Answer from the drawing. Dimensions are ordinates in mm from the lowest x, y and z of the part. Give positions to 0.01 mm unless a question says otherwise; leave off trailing zeros. Write each loop counter-clockwise with the first axis right and the second up, starting at its lowest first coordinate (ties: lowest second). Pieces come first, ordered by that corner, then holes.
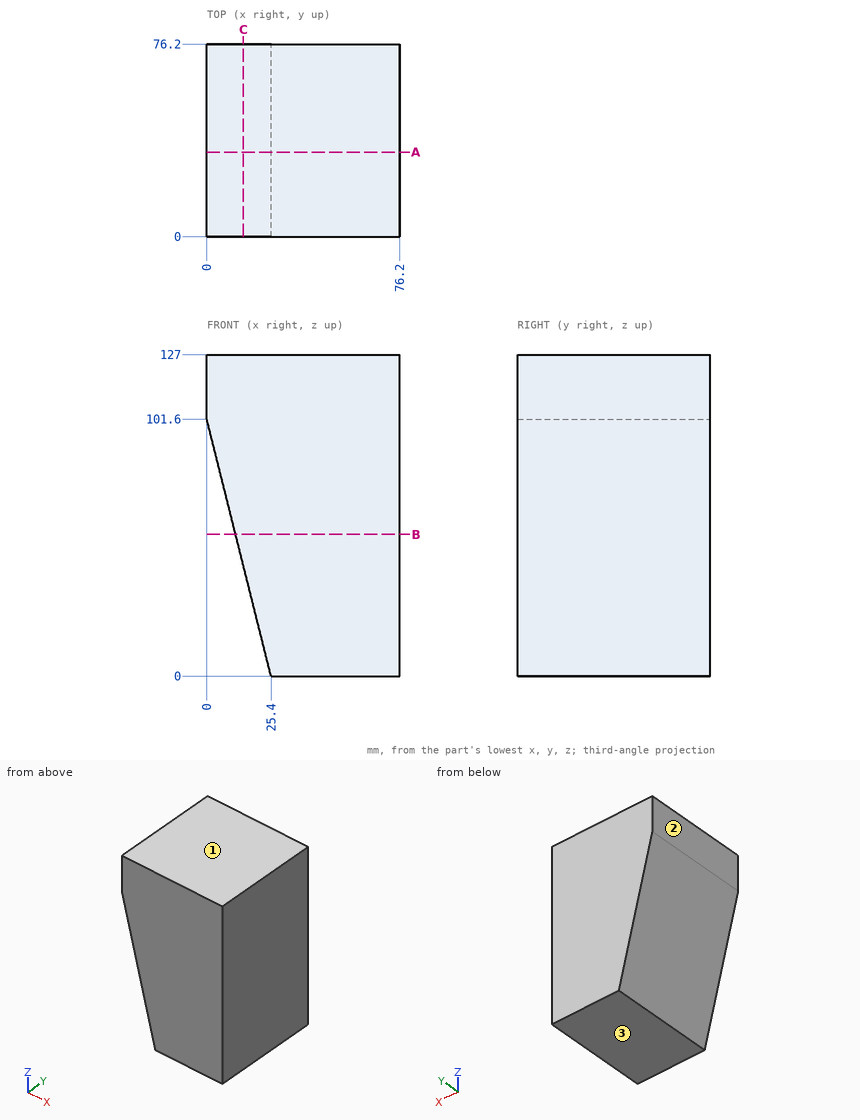
Item 1: A cutting plane is placed at B-B, the plane z = 56. Give the vertices of the cut face in (x, y), plus the area to 3 significant figures.
Conclusion:
outline: (11.4, 0) - (76.2, 0) - (76.2, 76.2) - (11.4, 76.2) - close
area: 4,940 mm2
Item 2: A cutting plane is placed at A-A, the plane y = 33.5. Give the vertices of the cut face in (x, z), plus the area to 3 significant figures.
Conclusion:
outline: (0, 101.6) - (25.4, 0) - (76.2, 0) - (76.2, 127) - (0, 127) - close
area: 8,390 mm2
Item 3: Determine the mould class of the marked faces 1, 2 and 3 for opening direction Z: pulls with the +Z half, pulls with the -Z half, needs draft (parallel to the pull), parting line crosses it, or undercut.
Conclusion:
face 1: pulls with the +Z half
face 2: needs draft
face 3: pulls with the -Z half
Item 4: Consider probe 1 along X at (y, z) = (49.5, 21.5) (3 decimals); probe 2 along X at (y, z) = (64, 41). Determine where each line is inside the solid, lowest interval first.
Conclusion:
probe 1: x = 20.025 to 76.2
probe 2: x = 15.15 to 76.2
Item 5: A cutting plane is placed at C-C, the plane x = 14.5. Give the vertices of the cut face in (y, z).
Conclusion:
outline: (0, 43.6) - (76.2, 43.6) - (76.2, 127) - (0, 127) - close
Item 6: Each of these flat-tipped pins is pushed along its axis until it touches: P1, Ø1, axis at y = 47, z = 38.5, coming from the -X side; P2, Ø12, axis at y = 41, z = 37, coming from the -X side. Where does it stop, or does it pass through?
Conclusion:
P1: stops at x = 15.65
P2: stops at x = 14.65
